The drawing under review shows one solid part. Ordinate dimensions are in mm from its lowest x, y, z. Round coordinates to 2 decimals unless told otherwise and drop trailing zeros. Order: outer loops, then holes, each group sorted by start corner. A loop starts at its lowest first (then second) coordinate and runs counter-clockwise, first axis right, second up. Notation, with made-up numbers: (40, 20.25) -> (57, 20.25) arc R14 cw to (57, 46.25) -> close; hole circle Ø11 at (32.5, 38). An arc over 180 degrees is marked (long way). Return JSON: item names as keys, results as strings. Group by question number.
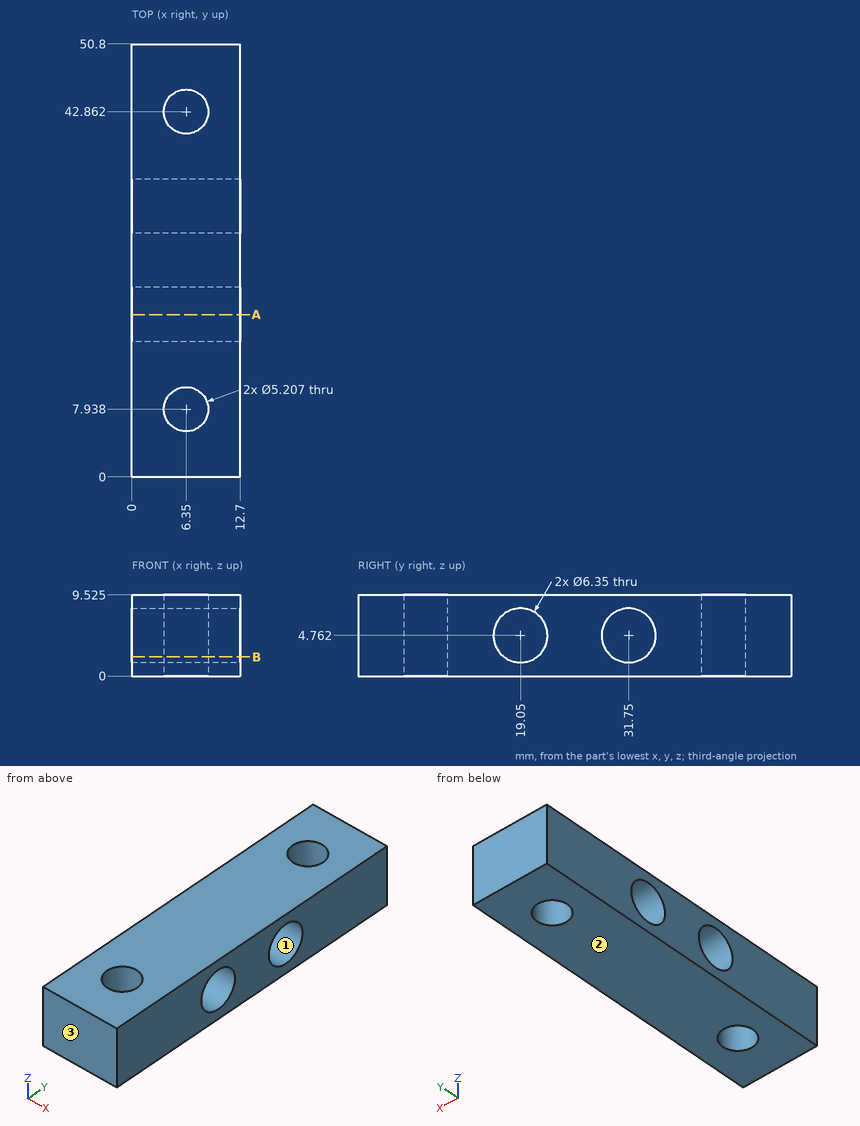
Item 1: Consider section B-B on z = 2.25. Give the number of separate pieces and of enclosed holes in the cut face, plus the area to 3 significant figures.
Item 2: Consider section A-A on y = 19.05. State the section outline as (x, z) points (1 decimal).
Item 3: Insertion check: pin 1 Ø5.5 at (y, z) = (19.05, 4.76) entering from +X. The pin has a flat end and moves straight along its axis. Give the tip position at first contact, or say it passes through.
Item 4: Wall thickness on line 1 along Y through (x, z) = (10, 5) (1 decimal); line 2 along Z through (x, y) = (4, 19.05) (1 decimal); line 3 along Y through (x, z) = (9.75, 3.5) (1 decimal): over which ranges is each line inside the solid? List them lowest first.
Item 5: The part is to be moulded in two halves that separate along Z. For the marked faces 1, 2 and 3, say which applies: +Z half, -Z half, draft (parallel to the pull), parting line (faces both ways), or undercut.
Values:
{
 "1": {"separate pieces": "3", "enclosed holes": "2", "area": "504 mm^2"},
 "2": {"outline": "(0, 0) -> (12.7, 0) -> (12.7, 1.6) -> (0, 1.6) -> close; (0, 7.9) -> (12.7, 7.9) -> (12.7, 9.5) -> (0, 9.5) -> close"},
 "3": {"pin 1": "through"},
 "4": {"line 1": "0 to 15.9, 22.2 to 28.6, 34.9 to 50.8", "line 2": "0 to 1.6, 7.9 to 9.5", "line 3": "0 to 16.1, 22 to 28.8, 34.7 to 50.8"},
 "5": {"face 1": "undercut", "face 2": "-Z half", "face 3": "draft"}
}
